Autodesk Inventor part; units mm, degrees
ref_plane "YZ Plane" through (0, 0, 0) normal (1, 0, 0) x (0, 1, 0)
ref_plane "XZ Plane" through (0, 0, 0) normal (0, 1, 0) x (-1, 0, 0)
ref_plane "XY Plane" through (0, 0, 0) normal (0, 0, 1) x (1, 0, 0)
sketch "Sketch1" plane through (0, 0, 0) normal (0, 1, 0) x (-1, 0, 0)
  line L0 (-63.5, 63.5) -> (63.5, 63.5)
  line L1 (63.5, 63.5) -> (63.5, -63.5)
  line L2 (63.5, -63.5) -> (-63.5, -63.5)
  line L3 (-63.5, -63.5) -> (-63.5, 63.5)
  line L4 (-63.5, 63.5) -> (63.5, -63.5) construction
  line L5 (63.5, 63.5) -> (-63.5, -63.5) construction
  line L6 (-69.85, 69.85) -> (69.85, 69.85)
  line L7 (69.85, 69.85) -> (69.85, -69.85)
  line L8 (69.85, -69.85) -> (-69.85, -69.85)
  line L9 (-69.85, -69.85) -> (-69.85, 69.85)
  line L10 (-69.85, 69.85) -> (69.85, -69.85) construction
  line L11 (69.85, 69.85) -> (-69.85, -69.85) construction
  point P0 (0, 0)
  dimension "d0" = 127
  dimension "d1" = 127
  dimension "d2" = 139.7
  dimension "d3" = 139.7
extrude "Extrusion1" add sketch "Sketch1" along normal blind 12.7
sketch "Sketch2" plane through (69.85, 0, -69.85) normal (0, 0, -1) x (-1, 0, 0)
  circle A0 centre (69.85, 6.35) radius 11.1125
  line L0 (0, 0) -> (0, 12.7) construction
  line L1 (0, 6.35) -> (69.85, 6.35) construction
  line L2 (69.85, 6.35) -> (139.7, 6.35) construction
  line L3 (139.7, 0) -> (139.7, 12.7) construction
  point P0 (69.85, 0)
  dimension "d6" = 22.225
extrude "Extrusion2" add sketch "Sketch2" against normal up to surface (6.35 mm away)
sketch "Sketch3" plane through (69.85, 0, -69.85) normal (0, 0, -1) x (-1, 0, 0)
  circle A0 centre (69.85, 6.35) radius 7.9375
  line L0 (0, 0) -> (0, 12.7) construction
  line L1 (0, 6.35) -> (69.85, 6.35) construction
  line L2 (69.85, 6.35) -> (139.7, 6.35) construction
  line L3 (139.7, 0) -> (139.7, 12.7) construction
  point P0 (69.85, 0)
  dimension "d9" = 15.875
extrude "Extrusion3" cut sketch "Sketch3" against normal up to next
sketch "Sketch4" plane through (-69.85, 0, 69.85) normal (0, 0, 1) x (1, 0, 0)
  circle A0 centre (69.85, 6.35) radius 11.1125
  line L0 (0, 0) -> (0, 12.7) construction
  line L1 (0, 6.35) -> (69.85, 6.35) construction
  line L2 (69.85, 6.35) -> (139.7, 6.35) construction
  line L3 (139.7, 0) -> (139.7, 12.7) construction
  point P0 (69.85, 0)
  dimension "d12" = 22.225
extrude "Extrusion4" add sketch "Sketch4" against normal up to surface (6.35 mm away)
sketch "Sketch5" plane through (-69.85, 0, 69.85) normal (0, 0, 1) x (1, 0, 0)
  circle A0 centre (69.85, 6.35) radius 6.35
  line L0 (0, 0) -> (0, 12.7) construction
  line L1 (0, 6.35) -> (69.85, 6.35) construction
  line L2 (69.85, 6.35) -> (139.7, 6.35) construction
  line L3 (139.7, 0) -> (139.7, 12.7) construction
  point P0 (69.85, 0)
  dimension "d15" = 12.7
extrude "Extrusion5" cut sketch "Sketch5" against normal up to next
properties part number "joystick_mount"
Build history of the part. All positions in model axes, mm. A direction names the side the tool comes from. Give positions to 0.01 mm unless a question says otherwise; leave off trailing zeros. Loops run counter-clockwise (first coordinate to the right, second up) from the corner with the lowest first, then second, coordinate; pieces in that order, holes last.
Item 1: Slice it at B-B, the plane y = 6.35. List the corners of the cut face in (x, z), and give its area (3 significant figures).
Answers follow:
outline: (-69.85, -69.85) - (-7.94, -69.85) - (-7.94, -63.5) - (-63.5, -63.5) - (-63.5, 63.5) - (-6.35, 63.5) - (-6.35, 69.85) - (-69.85, 69.85) - close; (6.35, 63.5) - (63.5, 63.5) - (63.5, -63.5) - (7.94, -63.5) - (7.94, -69.85) - (69.85, -69.85) - (69.85, 69.85) - (6.35, 69.85) - close
area: 3,210 mm2
Item 2: Slice it at A-A, the plane x = -17.5. List the corners of the cut face in (y, z), and give its area (3 significant figures).
Answers follow:
outline: (0, -69.85) - (12.7, -69.85) - (12.7, -63.5) - (0, -63.5) - close; (0, 63.5) - (12.7, 63.5) - (12.7, 69.85) - (0, 69.85) - close
area: 161 mm2
Item 3: Slice it at C-C, the plane x = 0. List the corners of the cut face in (y, z).
Answers follow:
outline: (-4.76, -69.85) - (-1.59, -69.85) - (-1.59, -63.5) - (-4.76, -63.5) - close; (-4.76, 63.5) - (0, 63.5) - (0, 69.85) - (-4.76, 69.85) - close; (12.7, 63.5) - (17.46, 63.5) - (17.46, 69.85) - (12.7, 69.85) - close; (14.29, -69.85) - (17.46, -69.85) - (17.46, -63.5) - (14.29, -63.5) - close
Item 4: Pull direction Y, two halves, no side cores. Call faces 1 (the face through (64, 12.7, 0)), 2 (the face through (5.85, 11.715, -66.719)), 3 (the face through (-0.827, 12.646, 66.719)), 4 (the face through (-0.15, -4.76, 66.72)): released by +Y, released by -Y, zero draft, split by the parting line, or undercut.
Answers follow:
face 1: released by +Y
face 2: undercut
face 3: undercut
face 4: released by -Y
Item 5: Which spindle directions (+Z, -Z, +X, -X, +Y, -Y) get a long thin tool onto all of the face, cutting with end or side? Do faces 5 (the face through (64, 0, 0)), 6 (the face through (-64, 12.7, 0)), 7 (the face through (-64, 0, 0)), 8 (the face through (-1, -1, 63.5)), 9 (the face through (0.15, -4.76, -66.72)). Say none if no direction does.
Answers follow:
face 5: +Z, -Z, +X, -Y
face 6: +Z, -Z, -X, +Y
face 7: +Z, -Z, -X, -Y
face 8: +Y, -Y
face 9: +Z, -Z, -Y
Item 6: Flat gauge pin, fed straight in: pin 1 (2 mm diameter, centred on y = 13.5, z = -20, fed in from +X). Where does the tip first touch, or does it go through?
Answers follow:
pin 1: stops at x = 69.85
Item 7: Drill centre lines: line 1 (X direction, y = 0.5, z = 47.5); line 2 (Y direction, x = 0, z = 66). Where is each one in solid material? Low to high.
Answers follow:
line 1: x = -69.85 to -63.5, 63.5 to 69.85
line 2: y = -4.76 to 0, 12.7 to 17.46
